Verification items for the finished model (mm, model axes). A direction names the side the tool comes from. Coordinates: 2 decimals unless noted, no trailing zeros. Order: outer loops, then holes, each group sorted by start corner. A loop starts at its lowest first (then second) coordinate and runs counter-clockwise, first axis right, second up. Notation, with made-up numbers: M 77,14.5 L 95,14.5 A11 ccw 95,25.5 Z; hole C 0,-38.5 d1. An arc over 180 degrees is marked long. Return JSON: item names as keys, results as strings.
```python
from build123d import *

# Parameters (mm, degrees)
SKETCH1_R           = 3.85
BOSS_EXTRUDE1_DEPTH = 2.5
SKETCH2_R           = 3.35
BOSS_EXTRUDE2_DEPTH = 0.75
CUT_EXTRUDE1_DEPTH  = 2.3


with BuildPart() as part:
    # Sketch1 → Boss-Extrude1 (new body)
    with BuildSketch(Plane(origin=(0, 0, 0), x_dir=(1, 0, 0), z_dir=(0, 1, 0))):
        with Locations(Location((0, 0, 0), (0, 0, 270))):
            Circle(SKETCH1_R)
    extrude(amount=BOSS_EXTRUDE1_DEPTH)

    # Sketch2 → Boss-Extrude2 (add)
    with BuildSketch(Plane(origin=(0, 2.5, 0), x_dir=(1, 0, 0), z_dir=(0, 1, 0))):
        with Locations(Location((0, 0, 0), (0, 0, 270))):
            Circle(SKETCH2_R)
    extrude(amount=BOSS_EXTRUDE2_DEPTH)

    # Sketch3 → Cut-Extrude1 (cut)
    with BuildSketch(Plane(origin=(0, 3.25, 0), x_dir=(1, 0, 0), z_dir=(0, 1, 0))):
        Polygon((-0.052616599, -2.612596145), (1.810178897, -1.884590005), (2.612596145, -0.052616599), (1.884590005, 1.810178897), (0.052616599, 2.612596145), (-1.810178897, 1.884590005), (-2.612596145, 0.052616599), (-1.884590005, -1.810178897), align=None)
    extrude(amount=-CUT_EXTRUDE1_DEPTH, mode=Mode.SUBTRACT)


solid = part.part
```
Q1. Cross-section at A-A, the plane y = 1.3. Record the boundary of the cut face in (x, z), and give its area (3 significant figures).
Values:
{"outline": "C 0,0 d7.7; hole M -2.61,-0.05 L -1.81,-1.88 L 0.05,-2.61 L 1.88,-1.81 L 2.61,0.05 L 1.81,1.88 L -0.05,2.61 L -1.88,1.81 Z", "area": "27.3 mm^2"}
Q2. Cross-section at D-D, the plane y = 0.7. Record the boundary of the cut face in (x, z), and give its area (3 significant figures).
Values:
{"outline": "C 0,0 d7.7", "area": "46.6 mm^2"}
Q3. Draft check along Z on faces 1 (the face through (0.981, 2.116, -2.206)), 2 (the face through (0, 0, 0)), 3 (the face through (-2.038, 2.87, -2.658)). Enter one of: pulls with the +Z half, pulls with the -Z half, needs draft (parallel to the pull), parting line crosses it, or undercut.
Values:
{"face 1": "undercut", "face 2": "needs draft", "face 3": "parting line crosses it"}
Q4. Cross-section at C-C, the plane x = 1.5. Record the boundary of the cut face in (y, z).
Values:
{"outline": "M 0,-3.55 L 2.5,-3.55 L 2.5,-3 L 3.25,-3 L 3.25,-1.98 L 0.95,-1.98 L 0.95,2.01 L 3.25,2.01 L 3.25,3 L 2.5,3 L 2.5,3.55 L 0,3.55 Z"}
Q5. Cross-section at B-B, the plane z = 3. Record the boundary of the cut face in (x, y).
Values:
{"outline": "M -2.41,0 L 2.41,0 L 2.41,2.5 L 1.49,2.5 L 1.49,3.25 L -1.49,3.25 L -1.49,2.5 L -2.41,2.5 Z"}
Q6. Material ranges on line 1 along Y through (x, z) = (-1.75, 0.75); line 2 along Y through (x, z) = (-0.25, 3.75); line 3 along Z through (x, y) = (0.25, 1.55), recorded low to high.
Values:
{"line 1": "0 to 0.95", "line 2": "0 to 2.5", "line 3": "-3.84 to -2.53, 2.49 to 3.84"}
Q7. Tool access check on faces 4 (the face through (2, 3.25, -2)), 5 (the face through (2.206, 2.116, 0.981)). Record the directions out of +Z, -Z, +X, -X, +Y, -Y that give a thin tool (end or side, any length) a straight path to the whole face; none if there is none.
Values:
{"face 4": "+Z, -Z, +X, -X, +Y", "face 5": "+Y"}
Q8. Go/stop test with flat-tipped pins: pin 1 (2.5 mm diameter, centred on x = -0.5, z = -0.5, fed in from +Y); pin 2 (1.5 mm diameter, centred on x = -2.5, y = 1, fed in from +Z). Record where each tip stops, or that it passes through.
Values:
{"pin 1": "y = 0.95", "pin 2": "z = 3.43"}
